Read the model definition and answer for the solid it produces. Units are mm, in the model's axes. A direction names the side the tool comes from. Give positions to 0.01 mm unless a question says otherwise; leave off trailing zeros. Order: outer loops, then holes, each group sorted by start corner. A loop starts at its lowest first (then second) coordinate and runs counter-clockwise, first axis right, second up.
Autodesk Inventor part; units mm, degrees
ref_plane "YZ Plane" through (0, 0, 0) normal (1, 0, 0) x (0, 1, 0)
ref_plane "XZ Plane" through (0, 0, 0) normal (0, 1, 0) x (-1, 0, 0)
ref_plane "XY Plane" through (0, 0, 0) normal (0, 0, 1) x (1, 0, 0)
sketch "Sketch1" plane through (0, 0, 0) normal (0, 0, 1) x (1, 0, 0)
  line L0 (0, 0) -> (22, 0)
  line L1 (22, 0) -> (22, 42)
  line L2 (22, 42) -> (0, 42)
  line L3 (0, 42) -> (0, 0)
  dimension "d0" = 42
  dimension "d1" = 22
extrude "Extrusion1" add sketch "Sketch1" along normal blind 22
sketch "Sketch2" plane through (0, 0, 0) normal (-1, 0, 0) x (0, 0, 1)
  circle A0 centre (11, 5) radius 2.5
  line L0 (0, 42) -> (0, 0)
  line L1 (0, 0) -> (22, 0)
  dimension "d4" = 11
  dimension "d5" = 5
  dimension "d6" = 5
extrude "Extrusion2" add sketch "Sketch2" along normal blind 10
sketch "Sketch3" plane through (22, 0, 0) normal (1, 0, 0) x (0, 0, -1)
  circle A0 centre (-11, 36) radius 2.5
  line L0 (0, 42) -> (-22, 42)
  line L1 (0, 0) -> (0, 42)
  dimension "d9" = 5
  dimension "d10" = 6
  dimension "d11" = 11
extrude "Extrusion3" add sketch "Sketch3" along normal blind 10
sketch "Sketch4" plane through (0, 42, 0) normal (0, 1, 0) x (1, 0, 0)
  line L0 (1, -1) -> (21, -1)
  line L1 (21, -1) -> (21, -21)
  line L2 (21, -21) -> (1, -21)
  line L3 (1, -21) -> (1, -1)
  line L4 (0, 0) -> (0, -22)
  line L5 (22, 0) -> (0, 0)
  line L6 (22, 0) -> (22, -22)
  line L7 (22, -22) -> (0, -22)
  dimension "d14" = 1
  dimension "d15" = 1
  dimension "d16" = 1
  dimension "d17" = 1
extrude "Extrusion4" cut sketch "Sketch4" against normal blind 41 contours L0 L1 L2 L3
sketch "Sketch5" plane through (0, 0, 0) normal (-1, 0, 0) x (0, 0, 1)
  circle A0 centre (11, 21) radius 5
  line L0 (0, 42) -> (0, 0)
  line L1 (0, 0) -> (22, 0)
  dimension "d20" = 11
  dimension "d21" = 10
  dimension "d22" = 21
extrude "Extrusion5" cut sketch "Sketch5" against normal through all
sketch "Sketch6" plane through (0, 0, 0) normal (0, 0, -1) x (-1, 0, 0)
  circle A0 centre (-11, 21) radius 5
  line L0 (0, 0) -> (-22, 0)
  line L1 (0, 42) -> (0, 0)
  dimension "d25" = 21
  dimension "d26" = 11
  dimension "d27" = 10
extrude "Extrusion6" cut sketch "Sketch6" against normal up to surface (1 mm away)
sketch "Sketch7" plane through (-10, 5, 11) normal (-1, 0, 0) x (0, 0, 1)
  circle A0 centre (0, 0) radius 1.5
  circle A1 centre (0, 0) radius 2.5
  point P0 (-11, -5)
  dimension "d30" = 1
extrude "Extrusion7" cut sketch "Sketch7" against normal up to surface (11 mm away) contours A0
sketch "Sketch8" plane through (32, 36, 11) normal (1, 0, 0) x (0, 0, -1)
  circle A0 centre (0, 0) radius 1.5
  circle A1 centre (0, 0) radius 2.5
  point P0 (11, -36)
  dimension "d33" = 1
extrude "Extrusion8" cut sketch "Sketch8" against normal up to surface (11 mm away) contours A0
sketch "Sketch9" plane through (0, 0, 22) normal (0, 0, 1) x (1, 0, 0)
  line L0 (20.3, 42) -> (20.3, 1)
  line L1 (20.3, 1) -> (1.7, 1)
  line L2 (1.7, 1) -> (1.7, 42)
  line L3 (0, 42) -> (0, 0)
  line L4 (0, 0) -> (22, 0)
  line L5 (22, 42) -> (0, 42)
  line L6 (22, 42) -> (0, 42)
  line L7 (1.7, 42) -> (0, 42)
  line L8 (0, 42) -> (0, 0)
  line L9 (0, 42) -> (0, 0)
  line L10 (0, 0) -> (22, 0)
  line L11 (22, 0) -> (22, 42)
  line L12 (22, 0) -> (22, 42)
  line L13 (22, 0) -> (22, 42)
  line L14 (20.3, 42) -> (22, 42)
  point P0 (1.7, 42)
  dimension "d37" = 1.7
  dimension "d38" = 1
extrude "Extrusion9" add sketch "Sketch9" along normal blind 5 contours L5 L11 L4 L3 L2 L1 L0
sketch "Sketch10" plane through (0, 42, 0) normal (0, 1, 0) x (1, 0, 0)
  line L0 (20.5, -24.6) -> (1.5, -24.6)
  line L1 (1.5, -24.6) -> (1.5, -23)
  line L2 (1.5, -23) -> (20.5, -23)
  line L3 (20.5, -23) -> (20.5, -24.6)
  line L4 (0, 0) -> (0, -27)
  line L5 (20.3, -22) -> (1.7, -22)
  dimension "d41" = 19
  dimension "d42" = 1.6
  dimension "d43" = 1.5
  dimension "d44" = 1
extrude "Extrusion10" cut sketch "Sketch10" against normal blind 41.2
sketch "Sketch12" plane through (1.7, 1, 27) normal (1, 0, 0) x (0, 0, -1)
  line L0 (2.4, 41) -> (2.4, -0.2)
  line L1 (2.4, 39.39) -> (0.9, 39.39)
  line L2 (0.9, 39.39) -> (0.9, 29.74)
  line L3 (0.9, 29.74) -> (2.4, 29.74)
  line L4 (2.4, 29.74) -> (2.4, 39.39)
  line L5 (2.4, -0.2) -> (4, -0.2)
  point P0 (27, -1)
  point P1 (2.4, 29.74)
  dimension "d48" = 1.5
  dimension "d49" = 9.65
  dimension "d50" = 29.94
extrude "Extrusion11" cut sketch "Sketch12" along normal through all both and the other way through all
sketch "Sketch13" plane through (20.3, 1, 27) normal (-1, 0, 0) x (0, 0, 1)
  line L0 (-2.4, 39.39) -> (-2.4, 29.74)
  line L1 (-2.4, 39.39) -> (-0.9, 39.39)
  line L2 (-0.9, 39.39) -> (-0.9, 41)
  line L3 (-0.9, 41) -> (-2.4, 41)
  line L4 (-2.4, 41) -> (-2.4, 39.39)
  line L5 (-0.9, 39.39) -> (-0.9, 29.74)
  line L6 (-2.4, 41) -> (0, 41)
  point P0 (-27, -1)
extrude "Extrusion12" cut sketch "Sketch13" against normal up to surface (0.2 mm away)
sketch "Sketch14" plane through (1.7, 1, 27) normal (1, 0, 0) x (0, 0, -1)
  line L0 (2.4, 39.39) -> (2.4, 41)
  line L1 (2.4, 39.39) -> (0.9, 39.39)
  line L2 (0.9, 39.39) -> (0.9, 41)
  line L3 (0.9, 41) -> (2.4, 41)
  line L4 (2.4, 41) -> (2.4, 39.39)
  line L5 (0.9, 29.74) -> (0.9, 39.39)
  line L6 (2.4, 41) -> (0, 41)
  point P0 (27, -1)
extrude "Extrusion13" cut sketch "Sketch14" against normal up to surface (0.2 mm away)
sketch "Sketch15" plane through (0, 0, 0) normal (-1, 0, 0) x (0, 0, 1)
  line L0 (0, 42) -> (0, 0)
  line L1 (4, 29) -> (21, 29)
  line L2 (21, 13) -> (4, 13)
  line L3 (4, 13) -> (4, 29)
  line L4 (2, 31) -> (21, 31)
  line L5 (21, 11) -> (2, 11)
  line L6 (2, 11) -> (2, 31)
  line L7 (21, 13) -> (21, 11)
  line L8 (21, 29) -> (21, 31)
  circle A0 centre (11, 21) radius 5
  dimension "d70" = 17
  dimension "d71" = 16
  dimension "d72" = 2
  dimension "d73" = 2
  dimension "d74" = 8
  dimension "d75" = 7
extrude "Extrusion15" add sketch "Sketch15" along normal blind 3 contours L3 L2 L7 L5 L6 L4 L8 L1
sketch "Sketch16" plane through (0, 11, 21) normal (0, 0, 1) x (1, 0, 0)
  line L0 (0, 31) -> (0, -11)
  line L1 (-0.13, 1) -> (0, 1)
  line L2 (0, 1) -> (0, 19)
  line L3 (0, 19) -> (-0.13, 19)
  line L4 (-0.13, 19) -> (-0.13, 1)
  line L5 (0, 0) -> (-3, 0)
  point P0 (0, 1)
  dimension "d78" = 0.13
  dimension "d79" = 18
  dimension "d80" = 1
extrude "Extrusion16" cut sketch "Sketch16" against normal blind 18
sketch "Sketch17" plane through (22, 0, 0) normal (1, 0, 0) x (0, 0, -1)
  line L0 (-21, 31) -> (-2, 31)
  line L1 (-2, 31) -> (-2, 11)
  line L2 (-2, 11) -> (-21, 11)
  line L3 (-21, 29) -> (-4, 29)
  line L4 (-4, 29) -> (-4, 13)
  line L5 (-4, 13) -> (-21, 13)
  line L6 (-21, 29) -> (-21, 31)
  line L7 (-21, 13) -> (-21, 11)
  circle A0 centre (-11, 21) radius 5
  point P0 (0, 0)
  point P1 (0, 67.5888)
  dimension "d89" = 2
  dimension "d90" = 16
  dimension "d91" = 17
  dimension "d92" = 2
  dimension "d93" = 8
  dimension "d94" = 7
extrude "Extrusion17" add sketch "Sketch17" along normal blind 3 contours L0 L1 L2 L7 L5 L4 L3 L6
sketch "Sketch19" plane through (22, 29, 21) normal (0, 0, 1) x (1, 0, 0)
  line L0 (0, 2) -> (0, -18)
  line L1 (0, 1) -> (0.13, 1)
  line L2 (0.13, 1) -> (0.13, -17)
  line L3 (0.13, -17) -> (0, -17)
  line L4 (0, -17) -> (0, 1)
  line L5 (0, 2) -> (3, 2)
  point P0 (-22, -29)
  point P1 (0, -17)
  dimension "d105" = 0.13
  dimension "d106" = 18
  dimension "d107" = 1
extrude "Extrusion19" cut sketch "Sketch19" against normal blind 18
sketch "Sketch18" plane through (0, 0, 0) normal (0, 0, -1) x (-1, 0, 0)
  line L0 (-1, 31) -> (-1, 12)
  line L1 (-1, 12) -> (-21, 12)
  line L2 (-21, 12) -> (-21, 31)
  line L3 (-3, 31) -> (-3, 14)
  line L4 (-3, 14) -> (-19, 14)
  line L5 (-19, 14) -> (-19, 31)
  line L6 (-21, 31) -> (-19, 31)
  line L7 (-3, 31) -> (-1, 31)
  circle A0 centre (-11, 21) radius 5
  point P0 (0, 0)
  dimension "d97" = 16
  dimension "d98" = 2
  dimension "d99" = 17
  dimension "d100" = 2
  dimension "d101" = 8
  dimension "d102" = 7
properties part number "Measurement"
1) Consider L1, parallel to Y at x = 0.3, z = 11; L2, parallel to Y at x = -5, z = 11; L3, parallel to Z at x = 17, y = 8.5. Determine where each line is inside the solid, lowest interval first.
Final values:
L1: y = 0 to 3.5, 6.5 to 16, 26 to 42
L2: y = 2.5 to 3.5, 6.5 to 7.5
L3: z = 0 to 1, 21 to 22
2) The part is cut by section A-A on x = 11. Determine the outline of the cut face in (y, z), and give its area (3 significant figures).
Final values:
outline: (0, 0) - (16, 0) - (16, 1) - (1, 1) - (1, 21) - (42, 21) - (42, 22) - (1, 22) - (1, 23) - (0.8, 23) - (0.8, 24.6) - (1, 24.6) - (1, 27) - (0, 27) - close; (26, 0) - (42, 0) - (42, 1) - (26, 1) - close
area: 98.7 mm2
3) The part is cut by section C-C on y = 5. Determine the outline of the cut face in (x, z).
Final values:
outline: (-10, 8.5) - (0, 8.5) - (0, 0) - (22, 0) - (22, 27) - (20.3, 27) - (20.3, 24.6) - (20.5, 24.6) - (20.5, 23) - (20.3, 23) - (20.3, 22) - (1.7, 22) - (1.7, 23) - (1.5, 23) - (1.5, 24.6) - (1.7, 24.6) - (1.7, 27) - (0, 27) - (0, 13.5) - (-10, 13.5) - (-10, 12.5) - (1, 12.5) - (1, 21) - (21, 21) - (21, 1) - (1, 1) - (1, 9.5) - (-10, 9.5) - close
4) The part is cut by section B-B on y = 36. Count the separate pieces of the cut face and the enclosed holes in it, and give its area (3 significant figures).
Final values:
separate pieces: 3
enclosed holes: 0
area: 112 mm2
5) Given pin 1 (1.9 mm diameter, centred on y = 15, z = 25.5, fed in from +X); pin 2 (1.4 mm diameter, centred on x = 23, y = 21, fed in from +Z); pin 3 (2.5 mm diameter, centred on y = 23.5, z = 26.5, fed in from -X), each flat-ended and moving along its own axis, determine where each tip first touches the part or whether it passes through.
Final values:
pin 1: stops at x = 22
pin 2: stops at z = 4
pin 3: stops at x = 0
6) A tool of negligible diameter and unlimited length cuts with its end or side. For faces 4 (the face through (11.1, 1, 22.5)), 5 (the face through (23, 11, 11)), 6 (the face through (-2, 13, 13)), 7 (the face through (1, 40.39, 25)), from which of +Z, -Z, +X, -X, +Y, -Y can it reach the whole face along a straight path? Write none if from no direction.
Final values:
face 4: +Z, +Y
face 5: +Z, -Z, +X, -Y
face 6: +Z, -X
face 7: +X, -X
7) For a pull along X with two mould halves and no side action, classify faces 1 (the face through (24, 21, 4)), 2 (the face through (1, 26.3, 11.1)), 3 (the face through (32, 36, 9)) as released by +X, released by -X, zero draft, split by the parting line, or undercut.
Final values:
face 1: zero draft
face 2: undercut
face 3: released by +X
